```python
from build123d import *

# Parameters (mm, degrees)
SKETCH1_R           = 4.7625
SKETCH1_R_2         = 1.5875
BOSS_EXTRUDE1_DEPTH = 3.175


with BuildPart() as part:
    # Sketch1 → Boss-Extrude1 (new body)
    # profile 1 of 3: a face of its own
    with BuildSketch(Plane.XY):
        with BuildLine():
            Line((25.4, 4.7625), (0, 4.7625))
            ThreePointArc((0, 4.7625), (3.367596045, 3.367596045), (4.7625, 0))
            ThreePointArc((4.7625, 0), (3.367596045, -3.367596045), (0, -4.7625))
            Line((0, -4.7625), (25.4, -4.7625))
            ThreePointArc((25.4, -4.7625), (20.6375, 0), (25.4, 4.7625))
        make_face()
    # profile 2 of 3: a face of its own
    with BuildSketch(Plane.XY):
        Circle(SKETCH1_R)
        with Locations(Location((0, 0, 0), (0, 0, 180))):
            Circle(SKETCH1_R_2, mode=Mode.SUBTRACT)
    # profile 3 of 3: a face of its own
    with BuildSketch(Plane.XY):
        with Locations((25.4, 0)):
            Circle(SKETCH1_R)
        with Locations(Location((25.4, 0, 0), (0, 0, 180))):
            Circle(SKETCH1_R_2, mode=Mode.SUBTRACT)
    extrude(amount=BOSS_EXTRUDE1_DEPTH)


solid = part.part
```
Model file for the job. Use its own axes, mm. Coordinates: 2 decimals unless noted, no trailing zeros. Write each loop counter-clockwise with the first axis right and the second up, starting at its lowest first coordinate (ties: lowest second). Pieces come first, ordered by that corner, then holes. Notation, with made-up numbers: (-12.75, 60) - (20.25, 60) arc R18 cw to (20.25, 78) - close; hole circle Ø10 at (71, 11.25). An arc over 180 degrees is marked (long way). Use a Markdown table: item, result. Add a question column.
Item 1: Band-saw the part on A-A, the plane y = 0. Write the cut outline in (x, z) (1 decimal).
Item 2: Band-saw the part on D-D, the plane y = 2. Write the cut outline in (x, z) (3 decimals).
Item 3: Band-saw the part on C-C, the plane y = 4. Write the cut outline in (x, z) (3 decimals).
Item 4: Two-plate mould, pull along X, no slides. Class faces 1 (the face through (-0.73, 1.41, 1.57)), 2 (the face through (13, 4.762, 2)), 3 (the face through (30.16, -0.1, 1.57)): pulls with the +X half, pulls with the -X half, needs draft (parallel to the pull), parting line crosses it, or undercut.
Item 5: Band-saw the part on B-B, the plane z = 0.85. Write the cut outline in (x, y) (1 decimal), and give its area (3 significant figures).
Item 6: Drill centre lines: line 1 along Y through (x, z) = (25.4, 0.7); line 2 along X through (y, z) = (1, 0.3); line 3 along X through (y, z) = (2, 1.75). Where is each one in solid material? Low to high.
Item 7: Drop a flat-ended pin along its axis: pin 1 (1 mm diameter, centred on y = 2.5, z = 1, fed in from +X). Give the stop position or say it passes through.
A:
| question | item | result |
|---|---|---|
| 1 | outline | (-4.8, 0) - (-1.6, 0) - (-1.6, 3.2) - (-4.8, 3.2) - close; (1.6, 0) - (23.8, 0) - (23.8, 3.2) - (1.6, 3.2) - close; (27, 0) - (30.2, 0) - (30.2, 3.2) - (27, 3.2) - close |
| 2 | outline | (-4.322, 0) - (29.722, 0) - (29.722, 3.175) - (-4.322, 3.175) - close |
| 3 | outline | (-2.585, 0) - (27.985, 0) - (27.985, 3.175) - (-2.585, 3.175) - close |
| 4 | face 1 | undercut |
| 4 | face 2 | needs draft |
| 4 | face 3 | pulls with the +X half |
| 5 | outline | (0, -4.8) - (25.4, -4.8) arc R4.8 ccw to (25.4, 4.8) - (0, 4.8) arc R4.8 ccw to start; hole circle Ø3.2 at (0, 0); hole circle Ø3.2 at (25.4, 0) |
| 5 | area | 297 mm² |
| 6 | line 1 | y = -4.76 to -1.59, 1.59 to 4.76 |
| 6 | line 2 | x = -4.66 to -1.23, 1.23 to 24.17, 26.63 to 30.06 |
| 6 | line 3 | x = -4.32 to 29.72 |
| 7 | pin 1 | stops at x = 29.72 |
